```python
from build123d import *

# Parameters (mm, degrees)
BOSS_EXTRUDE1_DEPTH = 6.35
SKETCH2_R           = 2.54
CUT_EXTRUDE1_DEPTH  = 6.35


with BuildPart() as part:
    # Sketch1 → Boss-Extrude1 (new body)
    with BuildSketch(Plane(origin=(0, 0, 0), x_dir=(1, 0, 0), z_dir=(0, 1, 0))):
        Polygon((0, -42.037783588), (-42.037783588, 0), (-54.737783588, 0), (-54.737783588, -22.673132337), (-22.673132337, -54.737783588), (0, -54.737783588), align=None)
        Polygon((0, 42.037783588), (0, 54.737783588), (-22.673132337, 54.737783588), (-54.737783588, 22.673132337), (-54.737783588, 0), (-42.037783588, 0), align=None)
        Polygon((22.673132337, 54.737783588), (0, 54.737783588), (0, 42.037783588), (42.037783588, 0), (54.737783588, 0), (54.737783588, 22.673132337), align=None)
        Polygon((54.737783588, 0), (42.037783588, 0), (0, -42.037783588), (0, -54.737783588), (22.673132337, -54.737783588), (54.737783588, -22.673132337), align=None)
    extrude(amount=BOSS_EXTRUDE1_DEPTH)

    # Sketch2 → Cut-Extrude1 (cut)
    with BuildSketch(Plane(origin=(0, 6.35, 0), x_dir=(1, 0, 0), z_dir=(0, 1, 0))):
        with Locations((-49.349629916, 17.284978664)):
            Circle(SKETCH2_R)
        with Locations((-42.165425019, 10.100773767)):
            Circle(SKETCH2_R)
        with Locations((-49.349629916, -17.284978664)):
            Circle(SKETCH2_R)
        with Locations((-42.165425019, -10.100773767)):
            Circle(SKETCH2_R)
        with Locations((49.349629916, 17.284978664)):
            Circle(SKETCH2_R)
        with Locations((42.165425019, 10.100773767)):
            Circle(SKETCH2_R)
        with Locations((42.165425019, -10.100773767)):
            Circle(SKETCH2_R)
        with Locations((49.349629916, -17.284978664)):
            Circle(SKETCH2_R)
    extrude(amount=-CUT_EXTRUDE1_DEPTH, mode=Mode.SUBTRACT)


solid = part.part
```
Here's how the part is built. I have some questions about the finished solid (model axes, mm). A direction names the side the tool comes from. Coordinates: 2 decimals unless noted, no trailing zeros. Write each loop counter-clockwise with the first axis right and the second up, starting at its lowest first coordinate (ties: lowest second). Pieces come first, ordered by that corner, then holes. Notation, with made-up numbers: (17.25, 2) -> (30.25, 2) arc R26 ccw to (30.25, 27) -> close; hole circle Ø3 at (33.25, 65.5). An arc over 180 degrees is marked (long way). Use a Markdown table: item, result. Add a question column.
(1) If we section it at B-B, the plane z = -24: Write out the boundary of the cut face in (x, y), and give its area (3 significant figures).
(2) We'd pull the mould along Z, two halves only. Please class faces 3 (the cylindrical face through (44.59, 3.22, 9.34)), 4 (the flat face through (-38.93, 3.13, 38.48)), 5 (the flat face through (-38.48, 3.13, -38.93)): +Z half, -Z half, draft (parallel to the pull), parting line (faces both ways), or undercut.
(3) If we section it at A-A, the plane x = -34: Write out the boundary of the cut face in (y, z).
(4) For faces 1 (the flat face through (-21.313, 3.131, -20.725)), 2 (the flat face through (-54.738, 3, 0)), which set-ups out of +Z, -Z, +X, -X, +Y, -Y let a thin tool reach every point of the face, with its end or its side?
(5) Please list where these lines run through material, in increasing order: line 1 (X direction, y = 4.25, z = 9.5); line 2 (Z direction, x = -43, y = 1); line 3 (X direction, y = 3.75, z = -17).
(6) If we section it at C-C, the plane y = 5.25: State how many separate pieces and enclosed holes the cut face has, and give its area (3 significant figures).
Outcome:
| question | item | result |
|---|---|---|
| 1 | outline | (-53.41, 0) -> (-18.04, 0) -> (-18.04, 6.35) -> (-53.41, 6.35) -> close; (18.04, 0) -> (53.41, 0) -> (53.41, 6.35) -> (18.04, 6.35) -> close |
| 1 | area | 449 mm^2 |
| 2 | face 3 | undercut |
| 2 | face 4 | +Z half |
| 2 | face 5 | -Z half |
| 3 | outline | (0, -43.41) -> (6.35, -43.41) -> (6.35, -8.04) -> (0, -8.04) -> close; (0, 8.04) -> (6.35, 8.04) -> (6.35, 43.41) -> (0, 43.41) -> close |
| 4 | face 1 | +Y, -Y |
| 4 | face 2 | +Z, -Z, -X, +Y, -Y |
| 5 | line 1 | x = -54.74 to -44.63, -39.7 to -32.54, 32.54 to 39.7, 44.63 to 54.74 |
| 5 | line 2 | z = -34.41 to -12.5, -7.7 to 7.7, 12.5 to 34.41 |
| 5 | line 3 | x = -54.74 to -51.87, -46.83 to -25.04, 25.04 to 46.83, 51.87 to 54.74 |
| 6 | separate pieces | 1 |
| 6 | enclosed holes | 9 |
| 6 | area | 6,230 mm^2 |
